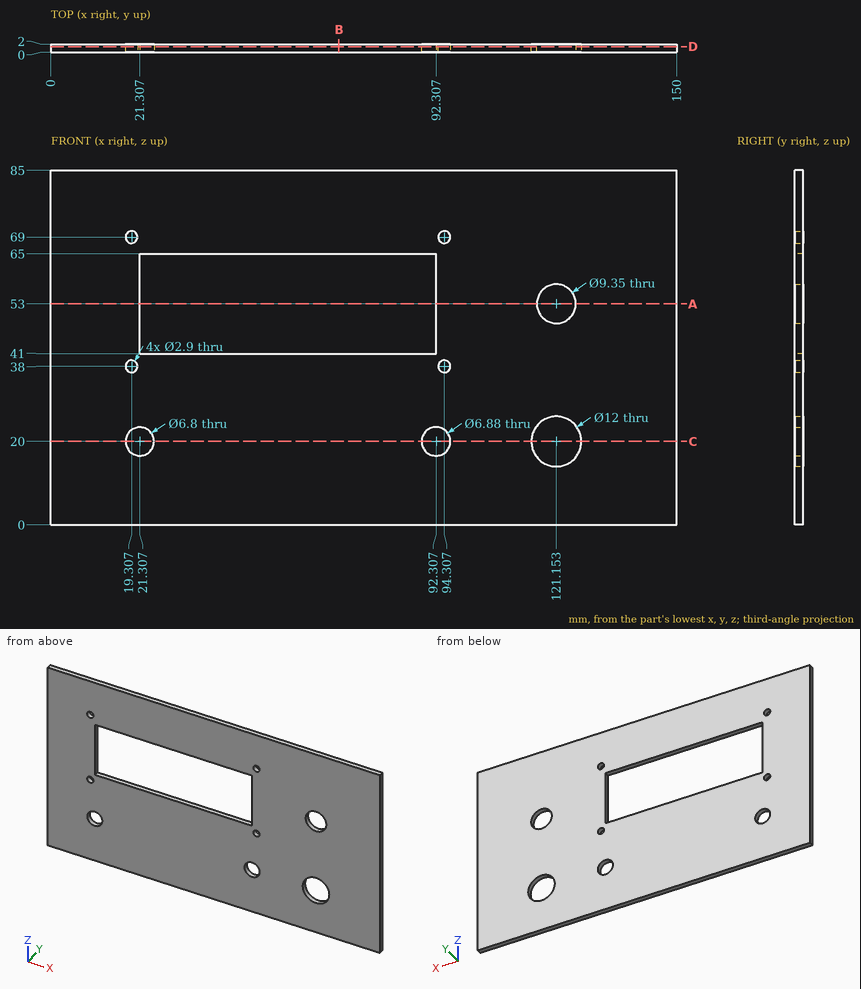
The figure shows three views and two pictorial views of one solid part (mm, origin at its lowest corner). Answer the questions. Give positions to 0.01 mm unless a question says otherwise; leave off trailing zeros. Write each loop counter-clockwise with the first axis right and the second up, starting at its lowest first coordinate (ties: lowest second). Pieces come first, ordered by that corner, then holes. Notation, with made-up numbers: (76.25, 2.5) - (90.25, 2.5) arc R21 ccw to (90.25, 28.5) - close; hole circle Ø1 at (0, -9.5). An arc over 180 degrees is marked (long way). Use one line per item in the form item = value. Start each with the question number.
1) Find section D-D on y = 1.35. Count the separate pieces of the cut face and the enclosed holes in it, plus the area to 3 significant figures.
2) Find section C-C on z = 20. Determine the outline of the cut face in (x, y).
3) Find section B-B on x = 69. Determine the outline of the cut face in (y, z), plus the area to 3 significant figures.
4) Consider line 1 along X through (y, z) = (0.8, 69); line 2 along X through (y, z) = (0.5, 45.5); line 3 along Z through (x, y) = (119, 1.5). Determine where each line is inside the solid, lowest interval first. Write a range as from..to.
5) Flat-ended cylindrical pins translate along their axes: pin 1 Ø5.5 at (x, z) = (21.31, 20) entering from -Y; pin 2 Ø1.5 at (x, z) = (21.5, 12) entering from -Y. Find the tip coordinate at first contact, or state that the pin passes through.
6) Find section A-A on z = 53. Determine the outline of the cut face in (x, y).
Geometry results:
q1.separate_pieces = 1
q1.enclosed_holes = 9
q1.area = 10,800 mm2
q2.outline = (0, 0) - (17.91, 0) - (17.91, 2) - (0, 2) - close; (24.71, 0) - (88.87, 0) - (88.87, 2) - (24.71, 2) - close; (95.75, 0) - (115.15, 0) - (115.15, 2) - (95.75, 2) - close; (127.15, 0) - (150, 0) - (150, 2) - (127.15, 2) - close
q3.outline = (0, 0) - (2, 0) - (2, 41) - (0, 41) - close; (0, 65) - (2, 65) - (2, 85) - (0, 85) - close
q3.area = 122 mm2
q4.line_1 = 0..17.86, 20.76..92.86, 95.76..150
q4.line_2 = 0..21.31, 92.31..150
q4.line_3 = 0..14.4, 25.6..48.85, 57.15..85
q5.pin_1 = through
q5.pin_2 = 0
q6.outline = (0, 0) - (21.31, 0) - (21.31, 2) - (0, 2) - close; (92.31, 0) - (116.48, 0) - (116.48, 2) - (92.31, 2) - close; (125.83, 0) - (150, 0) - (150, 2) - (125.83, 2) - close
